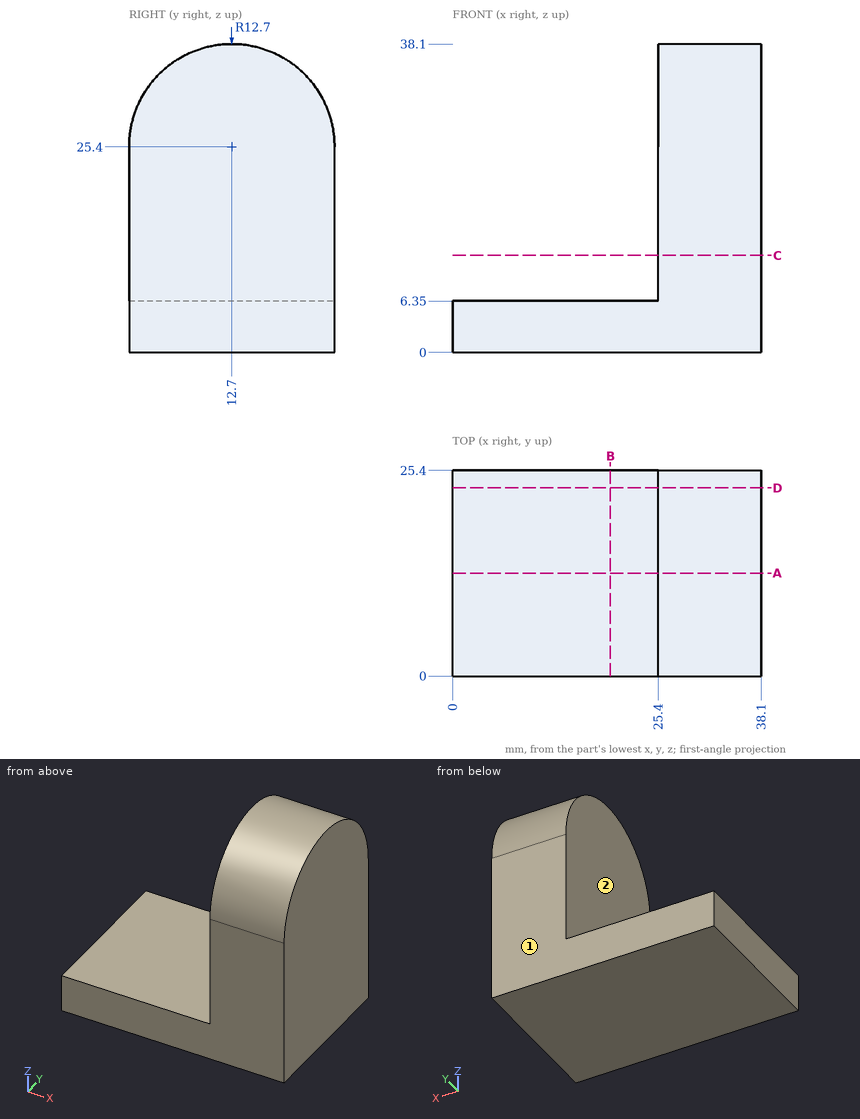
Geometry check sheet. Reference: drawing and pictorial views, mm from the part's lowest x, y, z. A direction names the side the tool comes from. Give positions to 0.01 mm unless a question says otherwise; leave off trailing zeros. Order: outer loops, then holes, each group sorted by start corner. A loop starts at its lowest first (then second) coordinate and runs counter-clockwise, first axis right, second up. Notation, with made-up numbers: (68, -39.75) -> (92, -39.75) arc R16 cw to (92, -34.75) -> close; hole circle Ø2 at (-2.5, -1.5). An arc over 180 degrees is marked (long way). Use CSV: the item, a comma, the result in double quotes. Start each with the question number.
1) Set-up check for the marked faces 1 and 2: record each of +Z, -Z, +X, -X, +Y, -Y from which the full face is reachable in a straight line by a thin tool's end or side.
2) Sectioned sample at B-B, the plane x = 19.5. Record the boundary of the cut face in (y, z).
3) Material ranges on line 1 (Z direction, x = 14, y = 22); line 2 (X direction, y = 13, z = 21.5); line 3 (Z direction, x = 35, y = 12.75), recorded low to high. Write a range as from..to.
4) Sectioned sample at C-C, the plane z = 12. Record the boundary of the cut face in (x, y).
5) Go/stop test with flat-tipped pins: P1, Ø6, axis at x = 21.5, y = 6, coming from the -Z side; P2, Ø4, axis at y = 7, z = 25, coming from the -X side; P3, Ø10, axis at x = 22.5, z = 32.5, coming from the -Y side; P4, Ø7.5, axis at x = 10, y = 15.5, coming from the +Z side. Record where each tip stops, or that it passes through.
6) Sectioned sample at A-A, the plane y = 12.7. Record the boundary of the cut face in (x, z), plus the area to 3 significant figures.
7) Sectioned sample at D-D, the plane y = 23.25. Record the boundary of the cut face in (x, z).
Recorded:
1,face 1,"+Z, -Z, +X, -X, +Y"
1,face 2,"+Z, -X, +Y, -Y"
2,outline,"(0, 0) -> (25.4, 0) -> (25.4, 6.35) -> (0, 6.35) -> close"
3,line 1,"0..6.35"
3,line 2,"25.4..38.1"
3,line 3,"0..38.1"
4,outline,"(25.4, 0) -> (38.1, 0) -> (38.1, 25.4) -> (25.4, 25.4) -> close"
5,P1,"z = 0"
5,P2,"x = 25.4"
5,P3,"y = 0.37"
5,P4,"z = 6.35"
6,outline,"(0, 0) -> (38.1, 0) -> (38.1, 38.1) -> (25.4, 38.1) -> (25.4, 6.35) -> (0, 6.35) -> close"
6,area,"645 mm2"
7,outline,"(0, 0) -> (38.1, 0) -> (38.1, 32.47) -> (25.4, 32.47) -> (25.4, 6.35) -> (0, 6.35) -> close"
